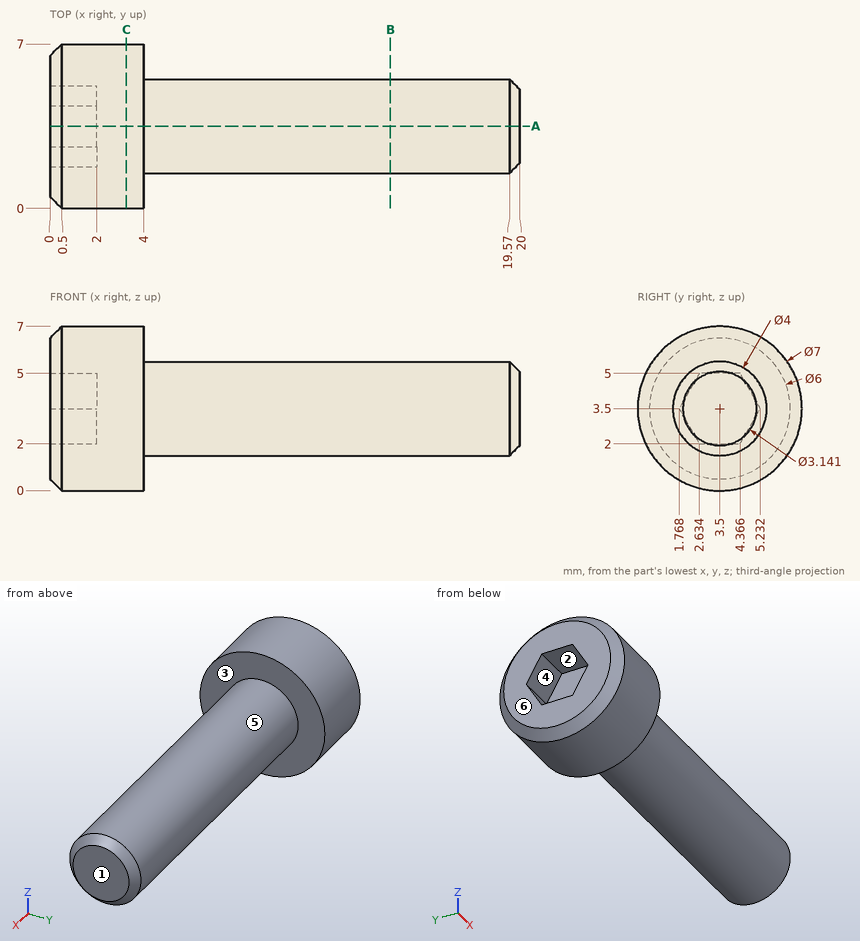
Could you check a few things on this drawing? It's one solid part, dimensions in mm from its lowest x, y, z. A direction names the side the tool comes from. Round coordinates to 2 decimals unless told otherwise and drop trailing zeros. Order: outer loops, then holes, each group sorted by start corner. A loop starts at its lowest first (then second) coordinate and runs counter-clockwise, first axis right, second up. Notation, with made-up numbers: M 30,33 L 71,33 A13 cw 71,47 Z; hole C -6,-38 d2. An arc over 180 degrees is marked long. One line per question, with ' | ' between items. Start each with the question number.
(1) Suppose I cut it at A-A on y = 3.5. List the corners of the cut face in (x, z) for me.
(2) Suppose I cut it at C-C on x = 3.25. List the corners of the cut face in (y, z) for me.
(3) For the marked faces 1, 2 and 3, which set-ups out of +Z, -Z, +X, -X, +Y, -Y let a thin tool reach every point of the face, with its end or its side?
(4) Suppose I cut it at B-B on x = 14.5. List the corners of the cut face in (y, z) for me.
(5) Please list where these lines run through material, in increasing order: line 1 along Z through (x, y) = (10.5, 2.5); line 2 along X through (y, z) = (5.5, 1.5); line 3 along X through (y, z) = (4.25, 4).
(6) For P1, Ø3, axis at x = 6.5, z = 1, coming from the +Y side; P2, Ø1.5, axis at y = 3.5, z = 3, coming from the -X side; P3, Ø4, axis at x = 14, y = 6, coming from the -Z side, each with a flat end and sliding along its axis, tell me the tip position at first contact or that it passes through.
(7) Thinking about a two-plate mould opening in Y: for the marked faces 4, 5 and 6, which applies, +Y half, -Y half, draft (parallel to the pull), parting line (faces both ways), or undercut?
Geometry results:
1) outline: M 0,0.5 L 0.5,0 L 4,0 L 4,1.5 L 19.57,1.5 L 20,1.93 L 20,5.07 L 19.57,5.5 L 4,5.5 L 4,7 L 0.5,7 L 0,6.5 L 0,5 L 2,5 L 2,2 L 0,2 Z
2) outline: C 3.5,3.5 d7
3) face 1: +Z, -Z, +X, +Y, -Y | face 2: -X | face 3: +X
4) outline: C 3.5,3.5 d4
5) line 1: 1.77 to 5.23 | line 2: 0 to 4 | line 3: 2 to 20
6) P1: y = 5.23 | P2: x = 2 | P3: z = 1.56
7) face 4: undercut | face 5: parting line | face 6: draft
